For this review, take the finished solid that the model builds, in its own axes (mm). Face numbers are marked on the shaded views. A direction names the side the tool comes from. Give positions to 0.01 mm unless a question says otherwise; leave off trailing zeros. Write each loop counter-clockwise with the first axis right and the second up, starting at its lowest first coordinate (ties: lowest second). Pieces come first, ordered by that corner, then holes. Notation, with made-up numbers: M 10.25,-26.75 L 45.25,-26.75 A14 cw 45.25,-16.75 Z; hole C -32.75,52.25 d8. An arc over 180 degrees is marked long. Use one line per item in the form item = value. Start each with the question number.
Q1. Mouldability with a two-part tool opening along Y and no side actions: class the marked faces 1, 2, 3 and 4 as released by +Y, released by -Y, zero draft, split by the parting line, or undercut.
Q2. Consider section B-B on x = 25. Write out the cut boundary in (y, z), and give its area (3 significant figures).
Q3. Consider section D-D on z = 29. Write out the cut boundary in (x, y), and give its area (3 significant figures).
Q4. Tool access review of the marked faces 5 and 6: name each direction out of +Z, -Z, +X, -X, +Y, -Y from which nothing blocks a thin tool from reaching the whole face with its end or side.
Q5. Clearance check with flat-ended pins moving along their axes: pin 1 Ø8 at (x, y) = (20.5, 10.5) entering from -Z; pin 2 Ø6 at (x, z) = (39.5, 32) entering from +Y; pin 3 Ø23.5 at (x, y) = (30, 23) entering from +Z; pin 4 Ø2.5 at (y, z) = (18, 2.5) entering from +X. State where each tip first meets the part, or that it passes through.
Q6. Consider section C-C on y = 25. Write out the cut boundary in (x, z).
Q7. For probe 1 along X at (y, z) = (43.15, 1.35); probe 2 along Y at (x, z) = (41.65, 3); probe 3 along Y at (x, z) = (41, 2), list the stretches that pass through material, from the lowest coordinate up. Write a range as [from, to].
Q8. Consider section A-A on y = 9.85. Write out the cut boundary in (x, z), and give its area (3 significant figures).
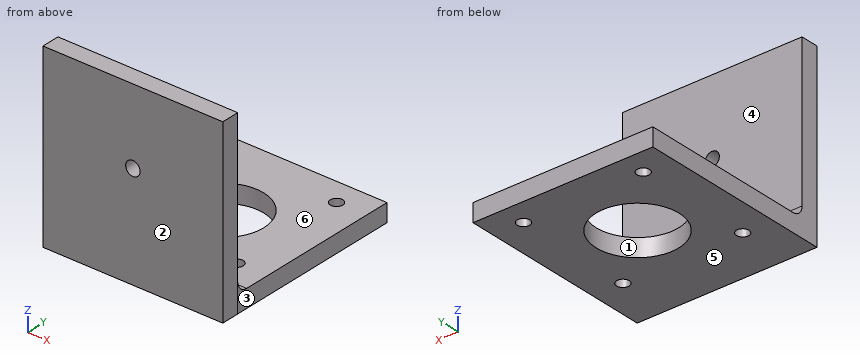
```python
from build123d import *

# Parameters (mm, degrees)
ESBO_O1_W                  = 50
ESBO_O1_H                  = 50
RESSALTO_EXTRUS_O1_DEPTH   = 5
ESBO_O2_R                  = 11.5
CORTE_EXTRUS_O1_DEPTH      = 8
CORTE_EXTRUS_O1_DEPTH_BACK = 14
ESBO_O3_W                  = 50.011024838
ESBO_O3_H                  = 5
RESSALTO_EXTRUS_O2_DEPTH   = 50
FILETE1_R                  = 3
ESBO_O4_R                  = 1.75
CORTE_EXTRUS_O2_DEPTH      = 11
ESBO_O5_R                  = 2
CORTE_EXTRUS_O4_DEPTH      = 14


with BuildPart() as part:
    # Esboço1 → Ressalto-extrusão1 (new body)
    with BuildSketch(Plane.XY):
        with Locations((25, 25)):
            Rectangle(ESBO_O1_W, ESBO_O1_H)
    extrude(amount=RESSALTO_EXTRUS_O1_DEPTH)

    # Esboço2 → Corte-extrusão1 (cut, two sides)
    with BuildSketch(Plane.XY) as corte_extrus_o1_sk:
        with Locations((25, 25)):
            Circle(ESBO_O2_R)
    extrude(amount=CORTE_EXTRUS_O1_DEPTH, mode=Mode.SUBTRACT)
    extrude(corte_extrus_o1_sk.sketch, amount=-CORTE_EXTRUS_O1_DEPTH_BACK, mode=Mode.SUBTRACT)

    # Esboço3 → Ressalto-extrusão2 (add)
    with BuildSketch(Plane.XY):
        with Locations((25.005512419, -2.5)):
            Rectangle(ESBO_O3_W, ESBO_O3_H)
    extrude(amount=RESSALTO_EXTRUS_O2_DEPTH)

    # Filete1
    filete1_edges = [part.edges().sort_by_distance(p)[0] for p in [
        (25, 0, 5),
    ]]
    fillet(filete1_edges, radius=FILETE1_R)

    # Esboço4 → Corte-extrusão2 (cut)
    with BuildSketch(Plane.XY):
        with Locations((8.35, 43.15)):
            Circle(ESBO_O4_R)
        with Locations((41.65, 43.15)):
            Circle(ESBO_O4_R)
        with Locations((41.65, 9.85)):
            Circle(ESBO_O4_R)
        with Locations((8.35, 9.85)):
            Circle(ESBO_O4_R)
    extrude(amount=CORTE_EXTRUS_O2_DEPTH, mode=Mode.SUBTRACT)

    # Esboço5 → Corte-extrusão4 (cut)
    with BuildSketch(Plane(origin=(0, 0, 0), x_dir=(1, 0, 0), z_dir=(0, 1, 0))):
        with Locations((25.002756209, -29)):
            Circle(ESBO_O5_R)
    extrude(amount=-CORTE_EXTRUS_O4_DEPTH, mode=Mode.SUBTRACT)


solid = part.part
```
Working result:
q1.face_1 = undercut
q1.face_2 = released by -Y
q1.face_3 = zero draft
q1.face_4 = released by +Y
q2.outline = M -5,0 L 13.5,0 L 13.5,5 L 3,5 A3 cw 0,8 L 0,27 L -5,27 Z; M -5,31 L 0,31 L 0,50 L -5,50 Z; M 36.5,0 L 50,0 L 50,5 L 36.5,5 Z
q2.area = 367 mm²
q3.outline = M 0,-5 L 23,-5 L 23,0 L 0,0 Z; M 27,-5 L 50.01,-5 L 50.01,0 L 27,0 Z
q3.area = 230 mm²
q4.face_5 = -Z, +X, -X, +Y, -Y
q4.face_6 = +Z, +X, -X, +Y
q5.pin_1 = 0
q5.pin_2 = 0
q5.pin_3 = 5
q5.pin_4 = 50
q6.outline = M 0,0 L 13.5,0 L 13.5,5 L 0,5 Z; M 36.5,0 L 50,0 L 50,5 L 36.5,5 Z
q7.probe_1 = [0, 6.6], [10.1, 39.9], [43.4, 50]
q7.probe_2 = [-5, 8.1], [11.6, 41.4], [44.9, 50]
q7.probe_3 = [-5, 8.23], [11.47, 41.53], [44.77, 50]
q8.outline = M 0,0 L 6.6,0 L 6.6,5 L 0,5 Z; M 10.1,0 L 39.9,0 L 39.9,5 L 10.1,5 Z; M 43.4,0 L 50,0 L 50,5 L 43.4,5 Z
q8.area = 215 mm²
